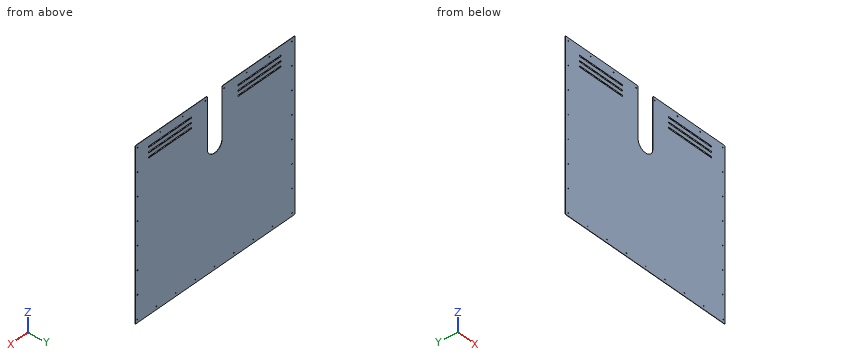
from build123d import *

# Parameters (mm, degrees)
F0_R     = 1.65
F1_DEPTH = 1


with BuildPart() as f1:
    # F0 (on Front) → F1 (new body)
    with BuildSketch(Plane.XZ):
        with BuildLine():
            ThreePointArc((120.203125, 125.020862), (90.203125, 95.020862), (60.203125, 125.020862))
            Line((60.203125, 125.020862), (60.203125, 307.955734))
            ThreePointArc((60.203125, 307.955734), (58.404687, 310.832687), (55.203125, 311.955734))
            Line((55.203125, 311.955734), (-235.296875, 311.955734))
            ThreePointArc((-235.296875, 311.955734), (-236.003982, 311.662841), (-236.296875, 310.955734))
            Line((-236.296875, 310.955734), (-236.296875, -313.044266))
            ThreePointArc((-236.296875, -313.044266), (-236.003982, -313.751373), (-235.296875, -314.044266))
            Line((-235.296875, -314.044266), (412.703125, -314.044266))
            ThreePointArc((412.703125, -314.044266), (413.410232, -313.751373), (413.703125, -313.044266))
            Line((413.703125, -313.044266), (413.703125, 310.955734))
            ThreePointArc((413.703125, 310.955734), (413.410232, 311.662841), (412.703125, 311.955734))
            Line((412.703125, 311.955734), (125.203125, 311.955734))
            ThreePointArc((125.203125, 311.955734), (122.001563, 310.832687), (120.203125, 307.955734))
            Line((120.203125, 307.955734), (120.203125, 125.020862))
        make_face()
        with Locations((-224.908055, -302.544266)):
            Circle(F0_R, mode=Mode.SUBTRACT)
        with Locations((-145.908055, -302.544266)):
            Circle(F0_R, mode=Mode.SUBTRACT)
        with Locations((-224.908055, -216.444266)):
            Circle(F0_R, mode=Mode.SUBTRACT)
        with Locations((-66.908055, -302.544266)):
            Circle(F0_R, mode=Mode.SUBTRACT)
        with Locations((12.091945, -302.544266)):
            Circle(F0_R, mode=Mode.SUBTRACT)
        with Locations((-224.908055, -130.344266)):
            Circle(F0_R, mode=Mode.SUBTRACT)
        with Locations((-224.908055, -44.244266)):
            Circle(F0_R, mode=Mode.SUBTRACT)
        with Locations((91.091945, -302.544266)):
            Circle(F0_R, mode=Mode.SUBTRACT)
        with Locations((170.091945, -302.544266)):
            Circle(F0_R, mode=Mode.SUBTRACT)
        with Locations((249.091945, -302.544266)):
            Circle(F0_R, mode=Mode.SUBTRACT)
        with Locations((328.091945, -302.544266)):
            Circle(F0_R, mode=Mode.SUBTRACT)
        with Locations((407.091945, -302.544266)):
            Circle(F0_R, mode=Mode.SUBTRACT)
        with Locations((405.262262, -216.076331)):
            Circle(F0_R, mode=Mode.SUBTRACT)
        with Locations((405.262262, -129.976331)):
            Circle(F0_R, mode=Mode.SUBTRACT)
        with Locations((405.262262, -43.876331)):
            Circle(F0_R, mode=Mode.SUBTRACT)
        with Locations((-224.908055, 41.855734)):
            Circle(F0_R, mode=Mode.SUBTRACT)
        with Locations((-224.908055, 127.955734)):
            Circle(F0_R, mode=Mode.SUBTRACT)
        with Locations((-224.908055, 214.055734)):
            Circle(F0_R, mode=Mode.SUBTRACT)
        with Locations((-224.908055, 300.155734)):
            Circle(F0_R, mode=Mode.SUBTRACT)
        with BuildLine():
            ThreePointArc((-179.546639, 240.567033), (-179.253746, 241.27414), (-178.546639, 241.567033))
            Line((-178.546639, 241.567033), (-5.546639, 241.567033))
            ThreePointArc((-5.546639, 241.567033), (-4.839533, 241.27414), (-4.546639, 240.567033))
            Line((-4.546639, 240.567033), (-4.546639, 237.567033))
            ThreePointArc((-4.546639, 237.567033), (-4.839533, 236.859927), (-5.546639, 236.567033))
            Line((-5.546639, 236.567033), (-178.546639, 236.567033))
            ThreePointArc((-178.546639, 236.567033), (-179.253746, 236.859927), (-179.546639, 237.567033))
            Line((-179.546639, 237.567033), (-179.546639, 240.567033))
        make_face(mode=Mode.SUBTRACT)
        with BuildLine():
            ThreePointArc((-179.546639, 258.567057), (-179.253745, 259.274164), (-178.546639, 259.567057))
            Line((-178.546639, 259.567057), (-5.546639, 259.567057))
            ThreePointArc((-5.546639, 259.567057), (-4.839532, 259.274164), (-4.546639, 258.567057))
            Line((-4.546639, 258.567057), (-4.546639, 255.567057))
            ThreePointArc((-4.546639, 255.567057), (-4.839532, 254.85995), (-5.546639, 254.567057))
            Line((-5.546639, 254.567057), (-178.546639, 254.567057))
            ThreePointArc((-178.546639, 254.567057), (-179.253745, 254.85995), (-179.546639, 255.567057))
            Line((-179.546639, 255.567057), (-179.546639, 258.567057))
        make_face(mode=Mode.SUBTRACT)
        with Locations((-132.608055, 300.155734)):
            Circle(F0_R, mode=Mode.SUBTRACT)
        with BuildLine():
            ThreePointArc((-179.546639, 277.571253), (-179.253745, 278.27836), (-178.546639, 278.571253))
            Line((-178.546639, 278.571253), (-5.546639, 278.571253))
            ThreePointArc((-5.546639, 278.571253), (-4.839532, 278.27836), (-4.546639, 277.571253))
            Line((-4.546639, 277.571253), (-4.546639, 274.571253))
            ThreePointArc((-4.546639, 274.571253), (-4.839532, 273.864146), (-5.546639, 273.571253))
            Line((-5.546639, 273.571253), (-178.546639, 273.571253))
            ThreePointArc((-178.546639, 273.571253), (-179.253745, 273.864146), (-179.546639, 274.571253))
            Line((-179.546639, 274.571253), (-179.546639, 277.571253))
        make_face(mode=Mode.SUBTRACT)
        with Locations((-40.308055, 300.155734)):
            Circle(F0_R, mode=Mode.SUBTRACT)
        with Locations((51.991945, 300.155734)):
            Circle(F0_R, mode=Mode.SUBTRACT)
        with Locations((405.262262, 42.223669)):
            Circle(F0_R, mode=Mode.SUBTRACT)
        with Locations((405.262262, 128.323669)):
            Circle(F0_R, mode=Mode.SUBTRACT)
        with Locations((128.362262, 300.523669)):
            Circle(F0_R, mode=Mode.SUBTRACT)
        with Locations((220.662262, 300.523669)):
            Circle(F0_R, mode=Mode.SUBTRACT)
        with Locations((405.262262, 214.423669)):
            Circle(F0_R, mode=Mode.SUBTRACT)
        with BuildLine():
            Line((184.952889, 237.567033), (184.952889, 240.567033))
            ThreePointArc((184.952889, 240.567033), (185.245783, 241.27414), (185.952889, 241.567033))
            Line((185.952889, 241.567033), (358.952889, 241.567033))
            ThreePointArc((358.952889, 241.567033), (359.659996, 241.27414), (359.952889, 240.567033))
            Line((359.952889, 240.567033), (359.952889, 237.567033))
            ThreePointArc((359.952889, 237.567033), (359.659996, 236.859927), (358.952889, 236.567033))
            Line((358.952889, 236.567033), (185.952889, 236.567033))
            ThreePointArc((185.952889, 236.567033), (185.245783, 236.859927), (184.952889, 237.567033))
        make_face(mode=Mode.SUBTRACT)
        with BuildLine():
            Line((184.952889, 255.567057), (184.952889, 258.567057))
            ThreePointArc((184.952889, 258.567057), (185.245782, 259.274164), (185.952889, 259.567057))
            Line((185.952889, 259.567057), (358.952889, 259.567057))
            ThreePointArc((358.952889, 259.567057), (359.659995, 259.274164), (359.952889, 258.567057))
            Line((359.952889, 258.567057), (359.952889, 255.567057))
            ThreePointArc((359.952889, 255.567057), (359.659995, 254.85995), (358.952889, 254.567057))
            Line((358.952889, 254.567057), (185.952889, 254.567057))
            ThreePointArc((185.952889, 254.567057), (185.245782, 254.85995), (184.952889, 255.567057))
        make_face(mode=Mode.SUBTRACT)
        with BuildLine():
            Line((184.952889, 274.571253), (184.952889, 277.571253))
            ThreePointArc((184.952889, 277.571253), (185.245782, 278.27836), (185.952889, 278.571253))
            Line((185.952889, 278.571253), (358.952889, 278.571253))
            ThreePointArc((358.952889, 278.571253), (359.659995, 278.27836), (359.952889, 277.571253))
            Line((359.952889, 277.571253), (359.952889, 274.571253))
            ThreePointArc((359.952889, 274.571253), (359.659995, 273.864146), (358.952889, 273.571253))
            Line((358.952889, 273.571253), (185.952889, 273.571253))
            ThreePointArc((185.952889, 273.571253), (185.245782, 273.864146), (184.952889, 274.571253))
        make_face(mode=Mode.SUBTRACT)
        with Locations((312.962262, 300.523669)):
            Circle(F0_R, mode=Mode.SUBTRACT)
        with Locations((405.262262, 300.523669)):
            Circle(F0_R, mode=Mode.SUBTRACT)
    extrude(amount=F1_DEPTH)


solid = f1.part
Geometry: final body of the model. Coordinates: model frame, mm. Give positions to 0.01 mm unless a question says otherwise; leave off trailing zeros. Write each loop counter-clockwise with the first axis right and the second up, starting at its lowest first coordinate (ties: lowest second). Pieces come first, ordered by that corner, then holes. Notation, with made-up numbers: M 80.25,5 L 96.25,5 A18 cw 96.25,19 Z; hole C 14,-9.5 d9. An arc over 180 degrees is marked long. Answer in a Markdown table with one row per item. Add a question column.
(1) Section B-B on y = -0.3. State how many separate pieces and enclosed holes the cut face has, and give its area (3 significant figures).
(2) Section A-A on x = -16. Return loops of the section in (y, z), and give its area (3 significant figures).
(3) Ray query, line 1 (X direction, y = -0.2, z = 238.5); line 2 (Z direction, x = -121, y = -0.55); line 3 (X direction, y = -0.7, z = 159.5). Return the intervals inside material, ascending.
Result set:
| question | item | result |
|---|---|---|
| 1 | separate pieces | 1 |
| 1 | enclosed holes | 35 |
| 1 | area | 389,000 mm^2 |
| 2 | outline | M -1,-314.04 L 0,-314.04 L 0,236.57 L -1,236.57 Z; M -1,241.57 L 0,241.57 L 0,254.57 L -1,254.57 Z; M -1,259.57 L 0,259.57 L 0,273.57 L -1,273.57 Z; M -1,278.57 L 0,278.57 L 0,311.96 L -1,311.96 Z |
| 2 | area | 611 mm^2 |
| 3 | line 1 | x = -236.3 to -179.55, -4.55 to 60.2, 120.2 to 184.95, 359.95 to 413.7 |
| 3 | line 2 | z = -314.04 to 236.57, 241.57 to 254.57, 259.57 to 273.57, 278.57 to 311.96 |
| 3 | line 3 | x = -236.3 to 60.2, 120.2 to 413.7 |
